Build history of the part. All positions in model axes, mm. Round coordinates to 2 decimals unless told otherwise and drop trailing zeros. Write each loop counter-clockwise with the first axis right and the second up, starting at its lowest first coordinate (ties: lowest second). Pieces come first, ordered by that corner, then holes. Notation, with made-up numbers: (60, 41.25) -> (76, 41.25) arc R15 cw to (76, 61.25) -> close; hole circle Ø9 at (-19, 59). An arc over 180 degrees is marked (long way). Return JSON: item names as keys, results as strings.
from build123d import *

# Parameters (mm, degrees)
F0_W     = 100
F0_H     = 70
F1_DEPTH = 4
F3_D     = 3.3
F4_D     = 3.2


with BuildPart() as f1:
    # F0 (on Top) → F1 (new body, symmetric)
    with BuildSketch(Plane.XY):
        Rectangle(F0_W, F0_H)
    extrude(amount=F1_DEPTH, both=True)

    # F3 (through all)
    with Locations(Plane.XY.offset(4)):
        with Locations((40, 25), (40, -25), (-40, -25), (-40, 25)):
            Hole(F3_D / 2)

    # F4 (through all)
    with Locations(Plane.XY.offset(4)):
        with Locations((0, 8), (0, -8)):
            Hole(F4_D / 2)


solid = f1.part
Q1. Wall check: L1, parallel to Y at x = -40, z = -1.5; L2, parallel to X at y = -24.5, z = 1.5. Give the ranges that are in metal, low to high.
Verdict:
{"L1": "y = -35 to -26.65, -23.35 to 23.35, 26.65 to 35", "L2": "x = -50 to -41.57, -38.43 to 38.43, 41.57 to 50"}
Q2. Saw through at A-A on x = 40. List the corners of the cut face in (y, z).
Verdict:
{"outline": "(-35, -4) -> (-26.65, -4) -> (-26.65, 4) -> (-35, 4) -> close; (-23.35, -4) -> (23.35, -4) -> (23.35, 4) -> (-23.35, 4) -> close; (26.65, -4) -> (35, -4) -> (35, 4) -> (26.65, 4) -> close"}
Q3. Pin check, flat tip, straight feed: pin 1 Ø5.5 at (x, y) = (-40, -25) entering from -Z. Stop position of the tip, or through.
Verdict:
{"pin 1": "stops at z = -4"}
Q4. Two-plate mould, pull along X, no slides. Class faces 1 (the flat face through (-50, 0, 0)), 2 (the flat face through (-1, 35, 0)), 3 (the cylindrical face through (0.35, -9.56, -0.06)): +X half, -X half, draft (parallel to the pull), parting line (faces both ways), or undercut.
Verdict:
{"face 1": "-X half", "face 2": "draft", "face 3": "undercut"}
Q5. Saw through at B-B on y = -25. List the corners of the cut face in (x, z).
Verdict:
{"outline": "(-50, -4) -> (-41.65, -4) -> (-41.65, 4) -> (-50, 4) -> close; (-38.35, -4) -> (38.35, -4) -> (38.35, 4) -> (-38.35, 4) -> close; (41.65, -4) -> (50, -4) -> (50, 4) -> (41.65, 4) -> close"}
